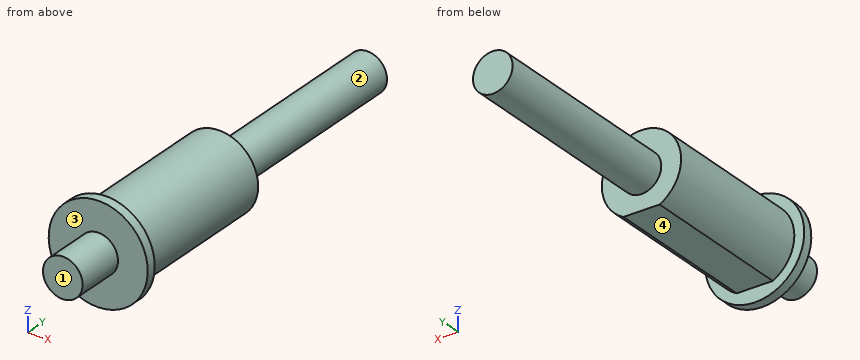
```python
from build123d import *

# Parameters (mm, degrees)
SKETCH_1_R      = 1
EXTRUDE_1_DEPTH = 21.5
EXTRUDE_START   = -2.5
SKETCH_2_R      = 2.5
SKETCH_2_R_2    = 1
EXTRUDE_2_DEPTH = 0.5
SKETCH_3_R      = 1
EXTRUDE_3_DEPTH = 8


with BuildPart() as part:
    # 草图1 → 凸台-拉伸1 (new body)
    with BuildSketch(Plane(origin=(0, 0, 0), x_dir=(1, 0, 0), z_dir=(0, 1, 0))):
        with Locations(Location((0, 0, 0), (0, 0, 270))):
            Circle(SKETCH_1_R)
    extrude(amount=EXTRUDE_1_DEPTH)

    # 草图2 → 凸台-拉伸2 (add)
    with BuildSketch(Plane.XZ.offset(EXTRUDE_START)):
        with Locations(Location((0, 0, 0), (0, 0, 270))):
            Circle(SKETCH_2_R)
        with Locations(Location((0, 0, 0), (0, 0, 270))):
            Circle(SKETCH_2_R_2, mode=Mode.SUBTRACT)
    extrude(amount=-EXTRUDE_2_DEPTH)

    # 草图3 → 凸台-拉伸3 (add)
    with BuildSketch(Plane(origin=(0, 3, 0), x_dir=(-1, 0, 0), z_dir=(0, 1, 0))):
        with BuildLine():
            Line((-0.911921049, -1.78), (0.911921049, -1.78))
            ThreePointArc((0.911921049, -1.78), (0, 2), (-0.911921049, -1.78))
        make_face()
        with Locations(Location((0, 0, 0), (0, 0, 270))):
            Circle(SKETCH_3_R, mode=Mode.SUBTRACT)
    extrude(amount=EXTRUDE_3_DEPTH)


solid = part.part
```
The listing builds one solid part. Answer for the finished solid, in the listing's coordinates (mm). Face numbers are marked on the shaded views. A direction names the side the tool comes from. Coordinates: 2 decimals unless noted, no trailing zeros. Write each loop counter-clockwise with the first axis right and the second up, starting at its lowest first coordinate (ties: lowest second). Pieces come first, ordered by that corner, then holes. Notation, with made-up numbers: M -27,17.5 L 25,17.5 A29 cw 25,40.5 Z; hole C 54.25,14 d11. An arc over 180 degrees is marked long. Use a Markdown table: item, result. Add a question column.
1. Given P1, Ø2, axis at x = 0, y = 8, coming from the -Z side; P2, Ø1, axis at x = 2, z = 0.5, coming from the -Y side, each flat-ended and moving along its own axis, determine where each tip first touches the part or whether it passes through.
2. Section D-D (z = 1.6) is taken. Give the vertices of the cut face in (x, y).
3. Section B-B (z = 0) is taken. Give the vertices of the cut face in (x, y), plus the area to 3 significant figures.
4. Straight lines are drawn through the part: line 1 along Y through (x, z) = (1.6, 1.4); line 2 along Y through (x, z) = (0.3, -1.6); line 3 along X through (y, z) = (12.25, -0.05). For each, find the intervals that lie inside material, in ascending order. Write a range as [from, to].
5. Section C-C (y = 18.75) is taken. Give the vertices of the cut face in (x, z).
6. Which of the six approach directions +Z, -Z, +X, -X, +Y, -Y give full straight-line access (tool end or side, diameter ignored) to the marked faces 1, 2, 3 and 4?
7. Section A-A (x = 0) is taken. Give the vertices of the cut face in (y, z), plus the area to 3 significant figures.
Data:
| question | item | result |
|---|---|---|
| 1 | P1 | stops at z = -1.78 |
| 1 | P2 | stops at y = 2.5 |
| 2 | outline | M -1.92,2.5 L 1.92,2.5 L 1.92,3 L 1.2,3 L 1.2,11 L -1.2,11 L -1.2,3 L -1.92,3 Z |
| 3 | outline | M -2.5,2.5 L -1,2.5 L -1,0 L 1,0 L 1,2.5 L 2.5,2.5 L 2.5,3 L 2,3 L 2,11 L 1,11 L 1,21.5 L -1,21.5 L -1,11 L -2,11 L -2,3 L -2.5,3 Z |
| 3 | area | 60.5 mm2 |
| 4 | line 1 | y = [2.5, 3] |
| 4 | line 2 | y = [2.5, 11] |
| 4 | line 3 | x = [-1, 1] |
| 5 | outline | C 0,0 d2 |
| 6 | face 1 | +Z, -Z, +X, -X, -Y |
| 6 | face 2 | +Y |
| 6 | face 3 | -Y |
| 6 | face 4 | -Z, +X, -X, +Y |
| 7 | outline | M 0,-1 L 2.5,-1 L 2.5,-2.5 L 3,-2.5 L 3,-1.78 L 11,-1.78 L 11,-1 L 21.5,-1 L 21.5,1 L 11,1 L 11,2 L 3,2 L 3,2.5 L 2.5,2.5 L 2.5,1 L 0,1 Z |
| 7 | area | 58.7 mm2 |
